from build123d import *

# Parameters (mm, degrees)
F1_DEPTH  = 6
F2_R      = 2.1
F3_DEPTH  = 25
F6_DEPTH  = 3
F7_R      = 1.5
F9_R      = 1.4
F10_DEPTH = 5


with BuildPart() as f1:
    # F0 (on Top) → F1 (new body, symmetric)
    with BuildSketch(Plane.XY):
        Polygon((12, -10), (12, 10), (8, 10), (8, -4), (0, -4), (-8, -4), (-8, 10), (-12, 10), (-12, -10), align=None)
    extrude(amount=F1_DEPTH, both=True)

    # F2 (on Right) → F3 (cut, symmetric)
    with BuildSketch(Plane.YZ):
        with Locations((5, 0)):
            Circle(F2_R)
    extrude(amount=F3_DEPTH, both=True, mode=Mode.SUBTRACT)

    # F5 (on offset) → F6 (cut)
    with BuildSketch(Plane.YZ.offset(12)):
        Polygon((5, -3.9259818305), (8.4, -1.9629909152), (8.4, 1.9629909152), (5, 3.9259818305), (1.6, 1.9629909152), (1.6, -1.9629909152), align=None)
    extrude(amount=-F6_DEPTH, mode=Mode.SUBTRACT)

    # F7
    f7_edges = [f1.edges().sort_by_distance(p)[0] for p in [
        (10, 10, -6),
        (10, 10, 6),
        (-10, 10, -6),
        (-10, 10, 6),
    ]]
    fillet(f7_edges, radius=F7_R)

    # F9 (on offset) → F10 (cut)
    with BuildSketch(Plane.XZ.offset(10)):
        Circle(F9_R)
    extrude(amount=-F10_DEPTH, mode=Mode.SUBTRACT)


solid = f1.part
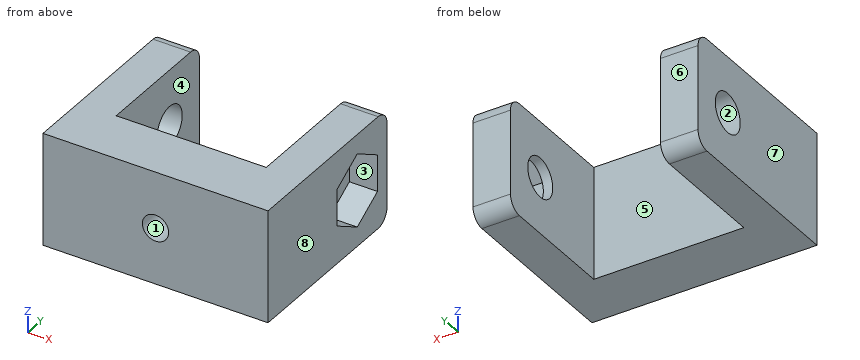
Can you work these out from the model? Positions are in its coordinate system, mm. Face numbers are marked on the shaded views. A direction names the side the tool comes from. Coordinates: 2 decimals unless noted, no trailing zeros. Write each loop counter-clockwise with the first axis right and the second up, starting at its lowest first coordinate (ties: lowest second). Pieces come first, ordered by that corner, then holes. Notation, with made-up numbers: (-15, -28) - (4, -28) arc R19 cw to (4, -3) - close; hole circle Ø5 at (29, 78.25). An arc over 180 degrees is marked (long way). Return JSON: item names as keys, results as strings. Group by question number.
Item 1: I'm going to push flat-ended pins straight in: pin 1 Ø5.5 at (y, z) = (5, -0.5) entering from +X; pin 2 Ø3 at (x, z) = (0.5, 0.5) entering from -Y; pin 3 Ø1 at (x, z) = (6.5, -1.5) entering from +Y; pin 4 Ø4 at (y, z) = (5, 0) entering from -X. Where does each tip first touch, or does it pass through?
Item 2: If we section it at C-C (y = 2): Write out the boundary of the cut face in (x, z).
Item 3: We'd pull the mould along X, two halves only. Please class the marked faces 5, 6, 7 and 8: pulls with the +X half, pulls with the -X half, needs draft (parallel to the pull), parting line crosses it, or undercut.
Item 4: If we section it at B-B (z = 0): Write out the boundary of the cut face in (x, y).
Item 5: Which directions (+Z, -Z, +X, -X, +Y, -Y) give clear straight access to the entire face, cutting with the end or side of a thin tool? Please do the marked faces 1, 2, 3 and 4.
Item 6: If we section it at A-A (x = -9.5): Write out the boundary of the cut face in (y, z), then the cut area to 3 significant figures.
Item 7: If we section it at D-D (x = 0): Write out the boundary of the cut face in (y, z), then the cut area to 3 significant figures.
Item 8: Please list where these lines run through material, in increasing order: probe 1 along X at (y, z) = (-3.5, 1); probe 2 along Y at (x, z) = (9.5, 0); probe 3 along Z at (x, y) = (8.3, 5).
Return value:
{
 "1": {"pin 1": "stops at x = 9", "pin 2": "stops at y = -10", "pin 3": "stops at y = -4", "pin 4": "passes through"},
 "2": {"outline": "(-12, -6) - (-8, -6) - (-8, 6) - (-12, 6) - close; (8, -6) - (12, -6) - (12, -2.19) - (9, -2.19) - (9, 2.19) - (12, 2.19) - (12, 6) - (8, 6) - close"},
 "3": {"face 5": "undercut", "face 6": "needs draft", "face 7": "pulls with the -X half", "face 8": "pulls with the +X half"},
 "4": {"outline": "(-12, -10) - (-1.4, -10) - (-1.4, -5) - (1.4, -5) - (1.4, -10) - (12, -10) - (12, 1.6) - (9, 1.6) - (9, 2.9) - (8, 2.9) - (8, -4) - (-8, -4) - (-8, 2.9) - (-12, 2.9) - close; (-12, 7.1) - (-8, 7.1) - (-8, 10) - (-12, 10) - close; (8, 7.1) - (9, 7.1) - (9, 8.4) - (12, 8.4) - (12, 10) - (8, 10) - close"},
 "5": {"face 1": "-Y", "face 2": "+X, -X", "face 3": "+X", "face 4": "+Z, -Z, +Y"},
 "6": {"outline": "(-10, -6) - (8.5, -6) arc R1.5 ccw to (10, -4.5) - (10, 4.5) arc R1.5 ccw to (8.5, 6) - (-10, 6) - close; hole circle Ø4.2 at (5, 0)", "area": "225 mm^2"},
 "7": {"outline": "(-10, -6) - (-4, -6) - (-4, 6) - (-10, 6) - (-10, 1.4) - (-5, 1.4) - (-5, -1.4) - (-10, -1.4) - close", "area": "58.0 mm^2"},
 "8": {"probe 1": "x = -12 to -8, 8 to 12", "probe 2": "y = -10 to 1.6, 8.4 to 10", "probe 3": "z = -6 to -2.1, 2.1 to 6"}
}
